The listing builds one solid part. Answer for the finished solid, in the listing's coordinates (mm). Give positions to 0.01 mm unless a question says otherwise; leave off trailing zeros. Write each loop counter-clockwise with the first axis right and the second up, starting at its lowest first coordinate (ties: lowest second). Pieces come first, ordered by that corner, then holes. Notation, with made-up numbers: (54.5, 0.25) -> (64.5, 0.25) arc R22 cw to (64.5, 12.25) -> close; hole circle Ø5 at (19, 68.5). An arc over 180 degrees is marked (long way). Put each result on its own line as item: value. Start each with the question number.
1) Flat-ended cylindrical pins translate along their axes: pin 1 Ø4 at (y, z) = (-354, -4.5) entering from +X; pin 2 Ø2 at (y, z) = (-284, -9.5) entering from +X; pin 3 Ø1.5 at (y, z) = (-362.5, -4.5) entering from -X. Find the tip coordinate at first contact, or state that the pin passes through.
2) Find the intervals of material crossed by line 1 along X through (y, z) = (-179.5, -4.5); line 2 along Z through (x, y) = (3.5, -61.5); line 3 along X through (y, z) = (-389, -8), in increasing order. Write a range as from..to.
3) A cutting plane is placed at A-A (y = -308). Write down the section's boundary in (x, z).
from build123d import *

# Parameters (mm, degrees)
F1_DEPTH    = 500.5
F2_R        = 4
F3_T1_DEPTH = 520.5
F3_T3_DEPTH = 519.2298334621
F4_T1_DEPTH = 525.22135955


# Not quite as in the source:
# - a fillet or chamfer that OpenCascade refuses, or shapes differently, is made with other operations: its cross-section is extruded or revolved along the edge and cut away or added


with BuildPart() as f1:
    # F0 (on Front) → F1 (new body)
    with BuildSketch(Plane.XZ):
        Polygon((9, 0), (0, 0), (-9, 0), (-9, -4), (-3, -4), (-3, -12), (3, -12), (3, -4), (9, -4), align=None)
    extrude(amount=F1_DEPTH)

    # F2
    f2_edges = [f1.edges().sort_by_distance(p)[0] for p in [
        (3, -250.25, -4),
        (-3, -250.25, -4),
    ]]
    fillet(f2_edges, radius=F2_R)

    # F3: fillet of radius 4 on 4 edges, made by hand

    # F3_s2 → F3_t1 (cut)
    with BuildSketch(Plane.XZ.offset(-10)):
        with BuildLine():
            ThreePointArc((-9, -4), (-7.8284271247, -1.1715728753), (-5, 0))
            Line((-5, 0), (-9, 0))
            Line((-9, 0), (-9, -4))
        make_face()
        with BuildLine():
            ThreePointArc((5, 0), (7.8284271247, -1.1715728753), (9, -4))
            Line((9, -4), (9, 0))
            Line((9, 0), (5, 0))
        make_face()
    extrude(amount=F3_T1_DEPTH, mode=Mode.SUBTRACT)

    # F3_s4 → F3_t3 (cut)
    with BuildSketch(Plane.XZ.offset(-9.364916731)):
        with BuildLine():
            ThreePointArc((-6, -4.1270166538), (-8.1622776602, -2.7035230504), (-9, -0.2540333076))
            Line((-9, -0.2540333076), (-9.4, -0.2540333076))
            Line((-9.4, -0.2540333076), (-9.4, -4))
            Line((-9.4, -4), (-9, -4.4))
            ThreePointArc((-9, -4.4), (-7, -4.4), (-6.1, -4.5143149884))
            Line((-6.1, -4.5143149884), (-6, -4.1270166538))
        make_face()
        with BuildLine():
            ThreePointArc((9, -0.2540333076), (8.1622776602, -2.7035230504), (6, -4.1270166538))
            Line((6, -4.1270166538), (6.1, -4.5143149884))
            ThreePointArc((6.1, -4.5143149884), (7, -4.4), (9, -4.4))
            Line((9, -4.4), (9.4, -4))
            Line((9.4, -4), (9.4, -0.2540333076))
            Line((9.4, -0.2540333076), (9, -0.2540333076))
        make_face()
    extrude(amount=F3_T3_DEPTH, mode=Mode.SUBTRACT)

    # F4: fillet of radius 5 on 2 edges, made by hand

    # F4_s2 → F4_t1 (cut)
    with BuildSketch(Plane.XZ.offset(-12.360679775)):
        with BuildLine():
            ThreePointArc((3.02476804, -7.5555555556), (1.3890614233, -10.7267799625), (-1.94427191, -12))
            Line((-1.94427191, -12), (-1.94427191, -12.5))
            Line((-1.94427191, -12.5), (3, -12.5))
            Line((3, -12.5), (3.5, -12))
            ThreePointArc((3.5, -12), (3.5, -8), (3.521672035, -7.6111111111))
            Line((3.521672035, -7.6111111111), (3.02476804, -7.5555555556))
        make_face()
        with BuildLine():
            ThreePointArc((1.94427191, -12), (-1.3890614233, -10.7267799625), (-3.02476804, -7.5555555556))
            Line((-3.02476804, -7.5555555556), (-3.521672035, -7.6111111111))
            ThreePointArc((-3.521672035, -7.6111111111), (-3.5, -8), (-3.5, -12))
            Line((-3.5, -12), (-3, -12.5))
            Line((-3, -12.5), (1.94427191, -12.5))
            Line((1.94427191, -12.5), (1.94427191, -12))
        make_face()
    extrude(amount=F4_T1_DEPTH, mode=Mode.SUBTRACT)


solid = f1.part
Reply:
1. pin 1: stops at x = 8.31
1. pin 2: stops at x = 2.83
1. pin 3: stops at x = -6.94
2. line 1: x = -5.06..5.06
2. line 2: z = -6.06..0
2. line 3: x = -2.95..2.95
3. outline: (-8.53, -2.13) arc R4 ccw to (-6, -4.13) arc R4 cw to (-3.02, -7.56) arc R5 ccw to (0, -11.61) arc R5 ccw to (3.02, -7.56) arc R4 cw to (6, -4.13) arc R4 ccw to (8.53, -2.13) arc R4 ccw to (5, 0) -> (-5, 0) arc R4 ccw to start
